from build123d import *

# Parameters (mm, degrees)
SKETCH1_W               = 170
SKETCH1_H               = 150
BOSS_EXTRUDE1_DEPTH     = 18
SKETCH2_R               = 65
CUT_EXTRUDE1_DEPTH      = 20
SHELL2_T                = -3
CUT_EXTRUDE2_DEPTH      = 20
CUT_EXTRUDE2_DEPTH_BACK = 20
SKETCH3_R               = 10
SKETCH4_R               = 2.5
CUT_EXTRUDE3_DEPTH      = 20
CHAMFER1_SIZE           = 5
SKETCH5_R               = 6
BOSS_EXTRUDE2_DEPTH     = 10


with BuildPart() as part:
    # Sketch1 → Boss-Extrude1 (new body)
    with BuildSketch(Plane.XY):
        Rectangle(SKETCH1_W, SKETCH1_H)
    extrude(amount=BOSS_EXTRUDE1_DEPTH)

    # Sketch2 → Cut-Extrude1 (cut)
    with BuildSketch(Plane(origin=(0, 0, 0), x_dir=(-1, 0, 0), z_dir=(0, 0, -1))):
        with Locations((-85, 75)):
            Circle(SKETCH2_R)
        with Locations((-85, -75)):
            Circle(SKETCH2_R)
        with Locations((65, 75)):
            Circle(SKETCH2_R)
        with Locations((65, -75)):
            Circle(SKETCH2_R)
    extrude(amount=-CUT_EXTRUDE1_DEPTH, mode=Mode.SUBTRACT)

    # Shell2
    shell2_openings = [part.faces().sort_by_distance(p)[0] for p in [
        (6.095773298, 0, 18),
    ]]
    offset(amount=SHELL2_T, openings=shell2_openings, kind=Kind.INTERSECTION)

    # Sketch3 → Cut-Extrude2 (cut, two sides: drawn at the far end of the back side and taken through both)
    with BuildSketch(Plane(origin=(0, 0, 0), x_dir=(1, 0, 0), z_dir=(0, 1, 0)).offset(-CUT_EXTRUDE2_DEPTH_BACK)):
        with Locations((-60, -18)):
            Circle(SKETCH3_R)
        with Locations((65, -18)):
            Circle(SKETCH3_R)
    extrude(amount=CUT_EXTRUDE2_DEPTH + CUT_EXTRUDE2_DEPTH_BACK, mode=Mode.SUBTRACT)

    # Sketch4 → Cut-Extrude3 (cut)
    with BuildSketch(Plane(origin=(0, 0, 0), x_dir=(-1, 0, 0), z_dir=(0, 0, -1))):
        with Locations((-10, -67)):
            Circle(SKETCH4_R)
        with Locations((-10, 67)):
            Circle(SKETCH4_R)
    extrude(amount=-CUT_EXTRUDE3_DEPTH, mode=Mode.SUBTRACT)

    # Chamfer1
    chamfer1_edges = [part.edges().sort_by_distance(p)[0] for p in [
        (-85, 0, 0),
        (85, 0, 0),
        (39.038059223, 29.038059223, 0),
        (39.038059223, -29.038059223, 0),
        (-26.757353648, 22.440509896, 0),
        (-26.757353648, -22.440509896, 0),
    ]]
    chamfer(chamfer1_edges, length=CHAMFER1_SIZE)

    # Sketch5 → Boss-Extrude2 (add)
    with BuildSketch(Plane(origin=(0, 0, 0), x_dir=(-1, 0, 0), z_dir=(0, 0, -1))):
        with Locations(Location((-22.5, 12.5, 0), (0, 0, 180))):
            Circle(SKETCH5_R)
        with Locations(Location((2.5, 12.5, 0), (0, 0, 180))):
            Circle(SKETCH5_R)
        with Locations(Location((2.5, -12.5, 0), (0, 0, 180))):
            Circle(SKETCH5_R)
        with Locations(Location((-22.5, -12.5, 0), (0, 0, 180))):
            Circle(SKETCH5_R)
    extrude(amount=BOSS_EXTRUDE2_DEPTH)


solid = part.part
Build history of the part. All positions in model axes, mm. A direction names the side the tool comes from. Coordinates: 2 decimals unless noted, no trailing zeros. Order: outer loops, then holes, each group sorted by start corner. A loop starts at its lowest first (then second) coordinate and runs counter-clockwise, first axis right, second up. Notation, with made-up numbers: (47.25, 18.25) - (86.25, 18.25) arc R6 cw to (86.25, 22.25) - close; hole circle Ø4 at (57.5, 0.5). An arc over 180 degrees is marked (long way). Write each question's results on one line, items separated by ' | '. Start each with the question number.
Item 1: Wall check: probe 1 along Y at (x, z) = (10, 1.95); probe 2 along X at (y, z) = (-6, 8.5); probe 3 along Y at (x, z) = (-34.5, 10.5). Give the ranges that are in metal, low to high. Write a range as [from, to].
Item 2: Flat gauge pins, fed straight in: pin 1 (4 mm diameter, centred on x = -9.5, z = -2.5, fed in from +Y); pin 2 (1.5 mm diameter, centred on x = 44, y = 2.5, fed in from -Z); pin 3 (1.5 mm diameter, centred on y = -30, z = 4.5, fed in from +X). Where does each tip first touch, or does it go through?
Item 3: Band-saw the part on B-B on z = 13.75. State how many separate pieces and enclosed holes the cut face has, and give its area (3 significant figures).
Item 4: Band-saw the part on A-A on x = 10. Write the cut outline in (y, z).
Item 5: Tool access for faces 1 (the face through (-60, -9, 8)), 2 (the face through (82, 0, 10)), 3 (the face through (18.08, 8.44, -4.93)): list every direction of +Z, -Z, +X, -X, +Y, -Y with a clear straight run to the whole face (end or side of a thin tool).
Numbers:
1) probe 1: [-75, -69.5], [-64.5, 64.5], [69.5, 75] | probe 2: [-85, -82], [82, 85] | probe 3: [-17.6, -14.22], [14.22, 17.6]
2) pin 1: y = 15.82 | pin 2: z = 0 | pin 3: x = 38.64
3) separate pieces: 4 | enclosed holes: 0 | area: 1,340 mm^2
4) outline: (-75, 0) - (-69.5, 0) - (-69.5, 3) - (-72, 3) - (-72, 18) - (-75, 18) - close; (-64.5, 0) - (64.5, 0) - (64.5, 3) - (-64.5, 3) - close; (69.5, 0) - (75, 0) - (75, 18) - (72, 18) - (72, 3) - (69.5, 3) - close
5) face 1: +Z, +Y, -Y | face 2: +Z | face 3: -Z
